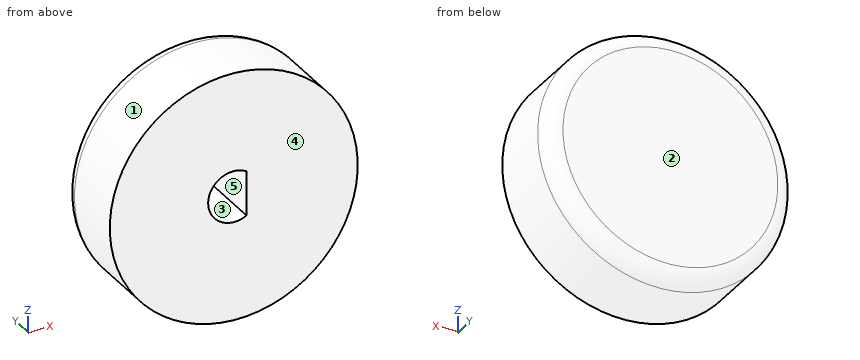
from build123d import *

# Parameters (mm, degrees)
CUT_EXTRUDE2_DEPTH = 7.5


with BuildPart() as part:
    # Sketch2 → Revolve1 (revolve)
    with BuildSketch(Plane(origin=(0, 0, 0), x_dir=(0, 0, -1), z_dir=(1, 0, 0))):
        with BuildLine():
            ThreePointArc((-15, 8), (-14.414213562, 9.414213562), (-13, 10))
            Line((-13, 10), (0, 10))
            Line((0, 10), (0, 0))
            Line((0, 0), (-15, 0))
            Line((-15, 0), (-15, 8))
        make_face()
    revolve(axis=Axis((0, 10, 0), (0, -1, 0)))

    # Sketch1 → Cut-Extrude2 (cut)
    with BuildSketch(Plane(origin=(0, 0, 0), x_dir=(1, 0, 0), z_dir=(0, 1, 0))):
        with BuildLine():
            Line((1.55, 2.684678752), (1.55, -2.684678752))
            ThreePointArc((1.55, -2.684678752), (-3.1, 0), (1.55, 2.684678752))
        make_face()
    extrude(amount=CUT_EXTRUDE2_DEPTH, mode=Mode.SUBTRACT)


solid = part.part
The listing builds one solid part. Answer for the finished solid, in the listing's coordinates (mm). Face numbers are marked on the shaded views. A direction names the side the tool comes from. Round coordinates to 2 decimals unless told otherwise and drop trailing zeros. Write each loop counter-clockwise with the first axis right and the second up, starting at its lowest first coordinate (ties: lowest second). Pieces come first, ordered by that corner, then holes. Notation, with made-up numbers: (-27.5, 7.5) - (5.5, 7.5) arc R30 ccw to (5.5, 30.5) - close; hole circle Ø9 at (1.25, 61). An arc over 180 degrees is marked (long way). Use a Markdown table: item, result. Add a question column.
1. Flat-ended cylindrical pins translate along their axes: P1, Ø5, axis at x = -10.5, y = 8.5, coming from the -Z side; P2, Ø7, axis at x = 0, z = 0, coming from the -Y side; P3, Ø1.4, axis at x = -1, z = 1.5, coming from the -Y side; P4, Ø1, axis at y = 2, z = -8, coming from the -X side. Find the tip coordinate at first contact, or state that the pin passes through.
2. For a pull along X with two mould halves and no side action, classify the marked faces 1, 2 and 3 as +X half, -X half, draft (parallel to the pull), parting line (faces both ways), or undercut.
3. Consider line 1 (X direction, y = 4.25, z = 0); line 2 (Z direction, x = 0, y = 3.5); line 3 (Z direction, x = 8.5, y = 2.25). Determine where each line is inside the solid, lowest interval first.
4. A tool of negligible diameter and unlimited length cuts with its end or side. For the marked faces 4 and 5, from which of +Z, -Z, +X, -X, +Y, -Y can it reach the whole face along a straight path? Write none if from no direction.
5. The part is cut by section A-A (z = 0). Write down the section's boundary in (x, y).
6. The part is cut by section C-C (y = 6). Write down the section's boundary in (x, z).
7. The part is cut by section B-B (x = 0). Write down the section's boundary in (y, z), and give its area (3 significant figures).
Reported:
| question | item | result |
|---|---|---|
| 1 | P1 | z = -12.67 |
| 1 | P2 | y = 0 |
| 1 | P3 | y = 7.5 |
| 1 | P4 | x = -12.99 |
| 2 | face 1 | parting line |
| 2 | face 2 | draft |
| 2 | face 3 | undercut |
| 3 | line 1 | -15 to -3.1, 1.55 to 15 |
| 3 | line 2 | -15 to -3.1, 3.1 to 15 |
| 3 | line 3 | -12.36 to 12.36 |
| 4 | face 4 | +Z, -Z, +X, -X, -Y |
| 4 | face 5 | -Y |
| 5 | outline | (-15, 0) - (-3.1, 0) - (-3.1, 7.5) - (1.55, 7.5) - (1.55, 0) - (15, 0) - (15, 8) arc R2 ccw to (13, 10) - (-13, 10) arc R2 ccw to (-15, 8) - close |
| 6 | outline | circle Ø30 at (0, 0); hole (1.55, -2.68) - (1.55, 2.68) arc R3.1 ccw (long way) to start |
| 7 | outline | (0, -15) - (8, -15) arc R2 ccw to (10, -13) - (10, 13) arc R2 ccw to (8, 15) - (0, 15) - (0, 3.1) - (7.5, 3.1) - (7.5, -3.1) - (0, -3.1) - close |
| 7 | area | 252 mm^2 |
